Source: CAD feature listing. Evaluate the final solid. Frame: model axes, mm. A direction names the side the tool comes from. Give positions to 0.01 mm unless a question says otherwise; leave off trailing zeros. Order: outer loops, then holes, each group sorted by start corner. A loop starts at its lowest first (then second) coordinate and runs counter-clockwise, first axis right, second up. Notation, with made-up numbers: M 54.25,17 L 107.25,17 A27 ccw 107.25,46 Z; hole C -5,26.25 d5. An arc over 180 degrees is marked long. Return JSON: item names as keys, results as strings.
from build123d import *

# Parameters (mm, degrees)
EXTRUDE_1_DEPTH = 796.883643365
OTHER_1_DEPTH   = 58


# Read off the part's stored shape, not the designer's step: Полость1
with BuildPart() as part:
    # Эскиз2 → Бобышка-Вытянуть1 (new body)
    with BuildSketch(Plane(origin=(0, 0, 0), x_dir=(0, 0, -1), z_dir=(1, 0, 0))):
        with BuildLine():
            Line((-58, -140), (-58, 0))
            Line((-58, 0), (0, 0))
            Line((0, 0), (0, -1.9))
            ThreePointArc((0, -1.9), (-0.878679656, -4.021320344), (-3, -4.9))
            Line((-3, -4.9), (-45.1, -4.9))
            ThreePointArc((-45.1, -4.9), (-50.756854249, -7.243145751), (-53.1, -12.9))
            Line((-53.1, -12.9), (-53.1, -127.1))
            ThreePointArc((-53.1, -127.1), (-50.756854249, -132.756854249), (-45.1, -135.1))
            Line((-45.1, -135.1), (-3, -135.1))
            ThreePointArc((-3, -135.1), (-0.878679656, -135.978679656), (0, -138.1))
            Line((0, -138.1), (0, -140))
            Line((0, -140), (-58, -140))
        make_face()
    extrude(amount=-EXTRUDE_1_DEPTH)

    # Полость1 outline → Полость1 (cut)
    with BuildSketch(Plane.XY):
        with BuildLine():
            Line((-796.883643365, -140), (-743.783643365, -140))
            Line((-743.783643365, -140), (-743.783643365, -138.1))
            ThreePointArc((-743.783643365, -138.1), (-744.662323022, -135.978679656), (-746.783643365, -135.1))
            Line((-746.783643365, -135.1), (-788.883643365, -135.1))
            ThreePointArc((-788.883643365, -135.1), (-794.540497615, -132.75685425), (-796.883643365, -127.1))
            Line((-796.883643365, -127.1), (-796.883643365, -140))
        make_face()
        with BuildLine():
            ThreePointArc((-796.883643365, -12.9), (-794.540497615, -7.24314575), (-788.883643365, -4.9))
            Line((-788.883643365, -4.9), (-746.783643365, -4.9))
            ThreePointArc((-746.783643365, -4.9), (-744.662323022, -4.021320343), (-743.783643365, -1.9))
            Line((-743.783643365, -1.9), (-743.783643365, 0))
            Line((-743.783643365, 0), (-796.883643365, 0))
            Line((-796.883643365, 0), (-796.883643365, -12.9))
        make_face()
    extrude(amount=OTHER_1_DEPTH, mode=Mode.SUBTRACT)

    # Зеркальное отражение1: part across plane


with BuildPart() as part_1:
    add(part.part)
    add(part.part.mirror(Plane(origin=(0, -1.9, 3), x_dir=(0, 0, 1), z_dir=(-1, 0, 0))))


solid = part_1.part
1. Section query A-A (z = 35). Return loops of the section in (x, y).
Evaluation:
{"outline": "M -746.78,-135.1 A3 cw -743.78,-138.1 L -743.78,-140 L 743.78,-140 L 743.78,-138.1 A3 cw 746.78,-135.1 Z; M -746.78,-4.9 L 746.78,-4.9 A3 cw 743.78,-1.9 L 743.78,0 L -743.78,0 L -743.78,-1.9 A3 cw Z"}
2. Section query B-B (x = -93.5). Return loops of the section in (y, z).
Evaluation:
{"outline": "M -140,0 L -138.1,0 A3 ccw -135.1,3 L -135.1,45.1 A8 cw -127.1,53.1 L -12.9,53.1 A8 cw -4.9,45.1 L -4.9,3 A3 ccw -1.9,0 L 0,0 L 0,58 L -140,58 Z"}
3. Set-up query: faces 1 (the face through (-10, -140, 29)), 2 (the face through (-11, -69, 53.1)). Return all of +Z, -Z, +X, -X, +Y, -Y with unobstructed straight access to the full face (end or side cutting, diameter ignored); none if empty.
Evaluation:
{"face 1": "+Z, -Z, +X, -X, -Y", "face 2": "-Z, +X, -X"}
4. Section query C-C (y = -52). Return loops of the section in (x, z).
Evaluation:
{"outline": "M -796.88,53.1 L 796.88,53.1 L 796.88,58 L -796.88,58 Z"}
5. Draft query along Y for faces 3 (the face through (-10, 0, 29)), 4 (the face through (-11, -71, 58)), 5 (the face through (-10, -4.9, 24)). Return one class per face: pulls with the +Y half, pulls with the -Y half, needs draft (parallel to the pull), parting line crosses it, or undercut.
Evaluation:
{"face 3": "pulls with the +Y half", "face 4": "needs draft", "face 5": "undercut"}
6. First-contact query: pin 1 (3 mm diameter, centred on x = -281.5, y = -35.5, fed in from -Z); pin 2 (4 mm diameter, centred on x = -769, z = 52, fed in from -Y); pin 3 (1.5 mm diameter, centred on y = -138.5, z = 26.5, fed in from -X). Flat tips, straight axial feed; report the tip coordinate or a pass-through.
Evaluation:
{"pin 1": "stops at z = 53.1", "pin 2": "stops at y = -135.1", "pin 3": "stops at x = -743.8"}
7. Ray query, probe 1 along Y at (x, z) = (-133.5, 22); probe 2 along Z at (x, y) = (-313, -82); probe 3 along Y at (x, z) = (-115, 48.5). Return the intervals inside material, ascending.
Evaluation:
{"probe 1": "y = -140 to -135.1, -4.9 to 0", "probe 2": "z = 53.1 to 58", "probe 3": "y = -140 to -134.34, -5.66 to 0"}
